For this review, take the finished solid that the model builds, in its own axes (mm). A direction names the side the tool comes from. Round coordinates to 2 decimals unless told otherwise and drop trailing zeros. Write each loop counter-clockwise with the first axis right and the second up, starting at its lowest first coordinate (ties: lowest second). Pieces come first, ordered by that corner, then holes. Notation, with made-up numbers: (80.25, -27) -> (111.25, -27) arc R22 cw to (111.25, 8) -> close; hole circle Ø6 at (10.5, -22). An arc over 180 degrees is marked (long way). Answer in a Markdown table with one row per item.
from build123d import *

# Parameters (mm, degrees)
SKETCH1_R           = 1.389
SKETCH1_R_2         = 0.889
BOSS_EXTRUDE1_DEPTH = 100
SKETCH2_R           = 2.5
BOSS_EXTRUDE2_DEPTH = 50
CUT_EXTRUDE1_DEPTH  = 1.5


with BuildPart() as part:
    # Sketch1 → Boss-Extrude1 (new body)
    with BuildSketch(Plane(origin=(0, 0, 0), x_dir=(1, 0, 0), z_dir=(0, 1, 0))):
        Circle(SKETCH1_R)
        Circle(SKETCH1_R_2, mode=Mode.SUBTRACT)
    extrude(amount=BOSS_EXTRUDE1_DEPTH)

    # Sketch2 → Boss-Extrude2 (add)
    with BuildSketch(Plane(origin=(0, 0, 0), x_dir=(1, 0, 0), z_dir=(0, 1, 0))):
        Circle(SKETCH2_R)
    extrude(amount=BOSS_EXTRUDE2_DEPTH)

    # Sketch3 → Cut-Extrude1 (cut)
    with BuildSketch(Plane(origin=(0, 100, 0), x_dir=(1, 0, 0), z_dir=(0, 1, 0))):
        Polygon((-2.121320344, 0), (0, 2.121320344), (0.901561146, 1.219759198), (-1.219759198, -0.901561146), align=None)
        Polygon((2.121320344, 0), (0, -2.121320344), (-0.901561146, -1.219759198), (1.219759198, 0.901561146), align=None)
    extrude(amount=-CUT_EXTRUDE1_DEPTH, mode=Mode.SUBTRACT)


solid = part.part
1) Consider section A-A on y = 45. State the section outline as (x, z) points.
Solved:
| item | result |
|---|---|
| outline | circle Ø5 at (0, 0) |
2) For line 1 (X direction, y = 84.5, z = 0); line 2 (Y direction, x = -1.4, z = -1.6), list the stretches that pass through material, from the lowest coordinate up. Write a range as [from, to].
Solved:
| item | result |
|---|---|
| line 1 | [-1.39, -0.89], [0.89, 1.39] |
| line 2 | [0, 50] |
3) Mouldability with a two-part tool opening along Z and no side actions: class faces 4 (the cylindrical face through (1.325, 74.65, -0.417)), 5 (the flat face through (-0.8, 98.5, -0.7)), 6 (the cylindrical face through (-0.19, 74.65, 0.87)) as pulls with the +Z half, pulls with the -Z half, needs draft (parallel to the pull), parting line crosses it, or undercut.
Solved:
| item | result |
|---|---|
| face 4 | parting line crosses it |
| face 5 | needs draft |
| face 6 | undercut |
4) For faces 1 (the flat face through (0.9, 98.5, 0.6)), 2 (the flat face through (0, 0, 0)), 3 (the flat face through (1.1, 50, 1.1)), list the 3-axis set-ups (+Z, -Z, +X, -X, +Y, -Y) from which the entire face can be reached by the end or side of a thin tool; tool diameter is ignored.
Solved:
| item | result |
|---|---|
| face 1 | +Z, +X, +Y |
| face 2 | +Z, -Z, +X, -X, -Y |
| face 3 | +Y |
5) Clearance check with flat-ended pins moving along their axes: pin 1 Ø2.5 at (x, z) = (-0.5, 0) entering from +Y; pin 2 Ø1 at (y, z) = (64.5, 0.5) entering from -X; pin 3 Ø1.5 at (x, y) = (1, 69.5) entering from -Z; pin 4 Ø1.4 at (x, z) = (0, 0) entering from +Y. State where each tip first meets the part, or that it passes through.
Solved:
| item | result |
|---|---|
| pin 1 | y = 100 |
| pin 2 | x = -1.39 |
| pin 3 | z = -1.37 |
| pin 4 | y = 50 |
